Verification items for the finished model (mm, model axes). Coordinates: 2 decimals unless noted, no trailing zeros. Loops run counter-clockwise (first coordinate to the right, second up) from the corner with the lowest first, then second, coordinate; pieces in that order, holes last.
Q1. Sectioned sample at C-C (y = -58). Enter the section's corners in (x, z).
Q2. Sectioned sample at A-A (z = 1767). Enter the section's corners in (x, y).
Q3. Go/stop test with flat-tipped pins: P1, Ø10, axis at x = -83, y = 46, coming from the +Z side; P2, Ø12, axis at x = -118, y = 39, coming from the -Z side. Record where each tip stops, or that it passes through.
Q4. Material ranges on probe 1 along Z at (x, y) = (21, 39.5), recorded low to high.
Q5. Sectioned sample at B-B (x = 11.5). Enter the section's corners in (y, z), then the cut area to 3 significant figures.
```python
from build123d import *

# Parameters (mm, degrees)
F0_W     = 381
F0_H     = 152.4
F1_DEPTH = 38.1
F2_R     = 6.726228
F4_DEPTH = 2000
F3_R     = 7.08762
F5_DEPTH = 2000


with BuildPart() as f1:
    # F0 (on Top) → F1 (new body)
    with BuildSketch(Plane.XY):
        Rectangle(F0_W, F0_H)
    extrude(amount=F1_DEPTH)

    # F2 (on Top) → F4 (join)
    with BuildSketch(Plane.XY):
        with Locations((-164.244667, 0)):
            Circle(F2_R)
    extrude(amount=F4_DEPTH)

    # F3 (on Top) → F5 (join)
    with BuildSketch(Plane.XY):
        with Locations((164.532065, 0)):
            Circle(F3_R)
    extrude(amount=F5_DEPTH)


solid = f1.part
```
Geometry check:
1. outline: (-190.5, 0) - (190.5, 0) - (190.5, 38.1) - (-190.5, 38.1) - close
2. outline: circle Ø13.45 at (-164.24, 0); circle Ø14.18 at (164.53, 0)
3. P1: stops at z = 38.1
3. P2: stops at z = 0
4. probe 1: z = 0 to 38.1
5. outline: (-76.2, 0) - (76.2, 0) - (76.2, 38.1) - (-76.2, 38.1) - close
5. area: 5,810 mm2
